Geometry: final body of the model. Coordinates: model frame, mm. A direction names the side the tool comes from. Round coordinates to 2 decimals unless told otherwise and drop trailing zeros. Write each loop counter-clockwise with the first axis right and the second up, starting at its lowest first coordinate (ties: lowest second). Pieces come first, ordered by that corner, then holes. Notation, with made-up numbers: (39, 83) -> (95, 83) arc R8 cw to (95, 90) -> close; hole circle Ø2 at (-11.75, 27.25). An arc over 180 degrees is marked (long way). Use one line per item in the form item = value. Start each with the question number.
1. Cut plane C-C, the plane x = -19. Return the cut outline in (y, z), plus the area to 3 significant figures.
2. Reachability of faces 4 (the face through (-19, 74, -25)), 5 (the face through (-19, 74, 22)) from +Z, -Z, +X, -X, +Y, -Y: full face, straight path, thin tool, end or side. Return the list, or none.
3. Pin query (flat end, axial travel): pin 1 Ø22 at (y, z) = (100.5, 10) entering from +X. Return the tip coordinate at first contact, or that it passes through.
4. Line query: L1, parallel to Y at x = -19, z = -22.9; L2, parallel to Z at x = -34.5, y = 71; L3, parallel to X at y = 55, z = 0.5. Output: solid intervals per line, ascending.
5. Cut plane B-B, the plane y = 130. Return the cut outline in (x, z).
6. Draft query along Y for faces 1 (the face through (-38, 0, -2)), 2 (the face through (0, 76, -23)), 3 (the face through (-15.786, 27.536, 23.479)). Return one class per face: pulls with the +Y half, pulls with the -Y half, needs draft (parallel to the pull), parting line crosses it, or undercut.
7. Cut plane A-A, the plane x = -5. Return the cut outline in (y, z).
8. Cut plane D-D, the plane z = 2. Return the cut outline in (x, y).
```python
from build123d import *

# Parameters (mm, degrees)
SKETCH_1_W          = 74
SKETCH_1_H          = 44
EXTRUDE_1_DEPTH     = 150
SKETCH_2_W          = 41.146480438
SKETCH_2_H          = 58.393385187
CUT_EXTRUDE_1_DEPTH = 151
SKETCH_3_R          = 4.05
CUT_EXTRUDE_2_DEPTH = 51


with BuildPart() as part:
    # Эскиз1 → Вытянуть-Тонкостенный1 (new body)
    with BuildSketch(Plane(origin=(0, 0, 0), x_dir=(1, 0, 0), z_dir=(0, 1, 0))):
        with BuildLine():
            Line((40, 22), (40, -22))
            ThreePointArc((40, -22), (39.121320344, -24.121320344), (37, -25))
            Line((37, -25), (-37, -25))
            ThreePointArc((-37, -25), (-39.121320344, -24.121320344), (-40, -22))
            Line((-40, -22), (-40, 22))
            ThreePointArc((-40, 22), (-39.121320344, 24.121320344), (-37, 25))
            Line((-37, 25), (37, 25))
            ThreePointArc((37, 25), (39.121320344, 24.121320344), (40, 22))
        make_face()
        Rectangle(SKETCH_1_W, SKETCH_1_H, mode=Mode.SUBTRACT)
    extrude(amount=EXTRUDE_1_DEPTH)

    # Эскиз2 → Вырез-Вытянуть1 (cut, through all)
    with BuildSketch(Plane(origin=(0, 150, 0), x_dir=(1, 0, 0), z_dir=(0, 1, 0))):
        with Locations((20.573240219, 1.776081122)):
            Rectangle(SKETCH_2_W, SKETCH_2_H)
    extrude(amount=-CUT_EXTRUDE_1_DEPTH, mode=Mode.SUBTRACT)

    # Эскиз3 → Вырез-Вытянуть2 (cut, through all)
    with BuildSketch(Plane(origin=(0, 0, -25), x_dir=(-1, 0, 0), z_dir=(0, 0, -1))):
        with Locations((19, 130)):
            Circle(SKETCH_3_R)
        with Locations((19, 30)):
            Circle(SKETCH_3_R)
    extrude(amount=-CUT_EXTRUDE_2_DEPTH, mode=Mode.SUBTRACT)


solid = part.part
```
Outcome:
q1.outline = (0, -25) -> (25.95, -25) -> (25.95, -22) -> (0, -22) -> close; (0, 22) -> (25.95, 22) -> (25.95, 25) -> (0, 25) -> close; (34.05, -25) -> (125.95, -25) -> (125.95, -22) -> (34.05, -22) -> close; (34.05, 22) -> (125.95, 22) -> (125.95, 25) -> (34.05, 25) -> close; (134.05, -25) -> (150, -25) -> (150, -22) -> (134.05, -22) -> close; (134.05, 22) -> (150, 22) -> (150, 25) -> (134.05, 25) -> close
q1.area = 803 mm^2
q2.face_4 = -Z, +X, -X, +Y, -Y
q2.face_5 = +X, +Y, -Y
q3.pin_1 = -37
q4.L1 = 0 to 25.95, 34.05 to 125.95, 134.05 to 150
q4.L2 = -25 to -22, 22 to 25
q4.L3 = -40 to -37
q5.outline = (-40, -22) arc R3 ccw to (-37, -25) -> (-23.05, -25) -> (-23.05, -22) -> (-37, -22) -> (-37, 22) -> (-23.05, 22) -> (-23.05, 25) -> (-37, 25) arc R3 ccw to (-40, 22) -> close; (-14.95, -25) -> (0, -25) -> (0, -22) -> (-14.95, -22) -> close; (-14.95, 22) -> (0, 22) -> (0, 25) -> (-14.95, 25) -> close
q6.face_1 = pulls with the -Y half
q6.face_2 = needs draft
q6.face_3 = undercut
q7.outline = (0, -25) -> (150, -25) -> (150, -22) -> (0, -22) -> close; (0, 22) -> (150, 22) -> (150, 25) -> (0, 25) -> close
q8.outline = (-40, 0) -> (-37, 0) -> (-37, 150) -> (-40, 150) -> close
